Geometry: final body of the model. Coordinates: model frame, mm. Face numbers are marked on the shaded views. A direction names the side the tool comes from. Give positions to 0.01 mm unless a question says otherwise; leave off trailing zeros. Loops run counter-clockwise (first coordinate to the right, second up) from the corner with the lowest first, then second, coordinate; pieces in that order, holes last.
1. Section A-A, the plane y = 46. Output: boundary loops of the cut face in (x, z).
2. Section C-C, the plane x = -32. Output: boundary loops of the cut face in (y, z).
3. Section D-D, the plane y = 107.5. Output: boundary loops of the cut face in (x, z).
4. Material intervals for line 1 along Z through (x, y) = (-13, 172.5); line 2 along X through (y, z) = (112.5, -81.5); line 3 along Z through (x, y) = (-80, 21), sorted ascending.
5. Section B-B, the plane z = 82.5. Output: boundary loops of the cut face in (x, y).
6. First-contact query: P1, Ø0.9, axis at x = -177, y = 159, coming from the -Z side; P2, Ø6, axis at x = -83.5, y = 184.5, coming from the +Z side; P3, Ø19.5, axis at y = 148, z = -138, coming from the +X side; P4, Ø10, axis at x = -91.5, z = 80.5, coming from the -Y side. Flat tips, straight axial feed; report the tip coordinate or a pass-through.
7. Access query for the marked faces 1, 2, 3 and 4. Directions: +Z, -Z, +X, -X, +Y, -Y. A direction counts if a zero-diameter tool reaches every point of the face in a straight line with its end or side. Return the directions, or none.
Autodesk Inventor part; units mm, degrees
ref_plane "YZ Plane" through (0, 0, 0) normal (1, 0, 0) x (0, 1, 0)
ref_plane "XZ Plane" through (0, 0, 0) normal (0, 1, 0) x (-1, 0, 0)
ref_plane "XY Plane" through (0, 0, 0) normal (0, 0, 1) x (1, 0, 0)
sketch "Sketch1" plane through (0, 0, 0) normal (0, 1, 0) x (-1, 0, 0)
  line L0 (0, 213.3361) -> (190.5, 213.3361)
  line L1 (190.5, 213.3361) -> (190.5, -167.6639)
  line L2 (190.5, -167.6639) -> (0, -167.6639)
  line L3 (0, -167.6639) -> (0, 213.3361)
  point P0 (0, 0)
  dimension "d0" = 190.5
  dimension "d1" = 381
extrude "Extrusion1" add sketch "Sketch1" along normal blind 12.7
sketch "Sketch2" plane through (0, 12.7, 0) normal (0, 1, 0) x (1, 0, 0)
  line L0 (0, -213.3361) -> (-190.5, -213.3361)
  line L1 (-190.5, -213.3361) -> (-190.5, 167.6639)
  line L2 (-190.5, 167.6639) -> (0, 167.6639)
  line L3 (0, 167.6639) -> (0, -213.3361)
  line L4 (-177.8, 154.9639) -> (-177.8, -200.6361)
  line L5 (-177.8, -200.6361) -> (-12.7, -200.6361)
  line L6 (-12.7, -200.6361) -> (-12.7, 154.9639)
  line L7 (-12.7, 154.9639) -> (-177.8, 154.9639)
  line L8 (-177.0062, -199.8424) -> (-177.0062, 154.1701)
  line L9 (-177.0062, 154.1701) -> (-13.4938, 154.1701)
  line L10 (-13.4938, 154.1701) -> (-13.4938, -199.8424)
  line L11 (-13.4938, -199.8424) -> (-177.0062, -199.8424)
  point P0 (0, 0)
  dimension "d4" = 12.7
  dimension "d5" = 0.7937
extrude "Extrusion2" add sketch "Sketch2" along normal blind 203.2 contours L7 L6 L5 L4
sketch "Sketch3" plane through (-12.7, 12.7, 200.6361) normal (1, 0, 0) x (0, 0, -1)
  line L0 (354.8062, 203.2) -> (265.9062, 203.2)
  line L1 (265.9062, 203.2) -> (265.9062, 0)
  line L2 (265.9062, 0) -> (354.8062, 0)
  line L3 (354.8062, 0) -> (354.8062, 203.2)
  line L4 (354.8062, 0) -> (0.7938, 0)
  line L5 (0.7938, 203.2) -> (89.6938, 203.2)
  line L6 (89.6938, 203.2) -> (89.6938, 0)
  line L7 (89.6938, 0) -> (0.7938, 0)
  line L8 (0.7938, 0) -> (0.7938, 203.2)
  line L9 (89.6938, 203.2) -> (265.9062, 203.2)
  line L10 (265.9062, 203.2) -> (265.9062, 0)
  line L11 (265.9062, 0) -> (89.6938, 0)
  line L12 (89.6938, 0) -> (89.6938, 203.2)
  point P0 (200.6361, -12.7)
  point P1 (0, 203.2)
  dimension "d9" = 88.9
  dimension "d10" = 88.9
extrude "Extrusion3" cut sketch "Sketch3" against normal blind 50.8 contours L1 L4 L6 L9
sketch "Sketch4" plane through (-177.0062, 12.7, 199.8424) normal (1, 0, 0) x (0, 0, -1)
  line L0 (265.1125, 0) -> (265.1125, 203.2)
  line L1 (88.9, 0) -> (265.1125, 0)
  line L2 (265.1125, 0) -> (265.1125, 50.8)
  line L3 (265.1125, 50.8) -> (88.9, 50.8)
  line L4 (88.9, 50.8) -> (88.9, 0)
  line L5 (88.9, 203.2) -> (265.1125, 203.2)
  line L6 (265.1125, 203.2) -> (265.1125, 114.3)
  line L7 (265.1125, 114.3) -> (88.9, 114.3)
  line L8 (88.9, 114.3) -> (88.9, 203.2)
  point P0 (199.8424, -12.7)
  dimension "d13" = 50.8
  dimension "d14" = 88.9
extrude "Extrusion4" cut sketch "Sketch4" against normal blind 50.8
sketch "Sketch5" plane through (-177.8, 12.7, 200.6361) normal (-1, 0, 0) x (0, 0, 1)
  line L0 (-265.9062, 114.3) -> (-265.9062, 203.2)
  line L1 (-355.6, 0) -> (-355.6, 203.2)
  line L2 (-368.3, 0) -> (12.7, 0)
  line L3 (-355.6, 203.2) -> (-330.2, 203.2)
  line L4 (-330.2, 203.2) -> (-330.2, 0)
  line L5 (-330.2, 0) -> (-355.6, 0)
  line L6 (-355.6, 0) -> (-355.6, 203.2)
  line L7 (-265.9062, 203.2) -> (-291.3062, 203.2)
  line L8 (-291.3062, 203.2) -> (-291.3062, 0)
  line L9 (-291.3062, 0) -> (-265.9062, 0)
  line L10 (-265.9062, 0) -> (-265.9062, 203.2)
  line L11 (-330.2, 203.2) -> (-291.3062, 203.2)
  line L12 (-291.3062, 203.2) -> (-291.3062, 0)
  line L13 (-291.3062, 0) -> (-330.2, 0)
  line L14 (-330.2, 0) -> (-330.2, 203.2)
  point P0 (-200.6361, -12.7)
  dimension "d17" = 89.6937
  dimension "d18" = 25.4
  dimension "d19" = 25.4
extrude "Extrusion5" cut sketch "Sketch5" against normal blind 25.4 contours L8 L2 L4 L11
sketch "Sketch6" plane through (-177.8, 12.7, 200.6361) normal (-1, 0, 0) x (0, 0, 1)
  line L0 (-89.6938, 114.3) -> (-265.9062, 114.3)
  line L1 (0, 0) -> (-89.6938, 0)
  line L2 (0, 203.2) -> (-25.4, 203.2)
  line L3 (-25.4, 203.2) -> (-25.4, 0)
  line L4 (-25.4, 0) -> (0, 0)
  line L5 (0, 0) -> (0, 203.2)
  line L6 (-89.6938, 203.2) -> (0, 203.2)
  line L7 (-89.6938, 0) -> (-64.2938, 0)
  line L8 (-64.2938, 0) -> (-64.2938, 203.2)
  line L9 (-64.2938, 203.2) -> (-89.6938, 203.2)
  line L10 (-89.6938, 203.2) -> (-89.6938, 0)
  line L11 (-64.2938, 203.2) -> (-25.4, 203.2)
  line L12 (-25.4, 203.2) -> (-25.4, 0)
  line L13 (-25.4, 0) -> (-64.2938, 0)
  line L14 (-64.2938, 0) -> (-64.2938, 203.2)
  line L15 (-64.2938, 203.2) -> (-25.4, 203.2)
  line L16 (-25.4, 203.2) -> (-25.4, 0)
  line L17 (-25.4, 0) -> (-64.2938, 0)
  line L18 (-64.2938, 0) -> (-64.2938, 203.2)
  point P0 (-200.6361, -12.7)
  dimension "d22" = 25.4
  dimension "d23" = 25.4
extrude "Extrusion6" cut sketch "Sketch6" against normal blind 25.4 contours L1 L8 L6 L3
properties part number "soccer_goal.ipj"
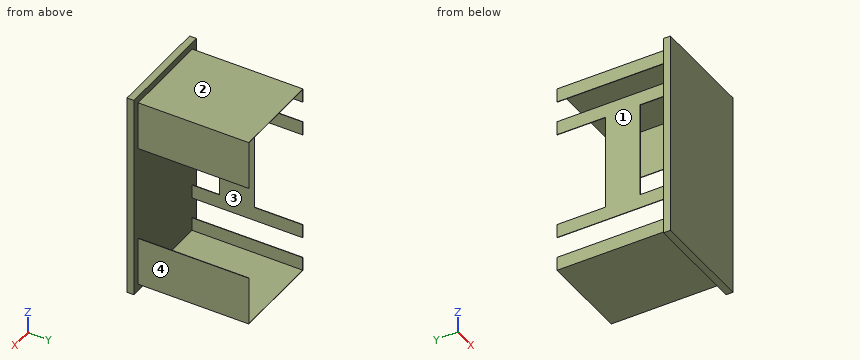
Answers below:
1. outline: (-177.8, -154.96) - (-12.7, -154.96) - (-12.7, -65.27) - (-13.49, -65.27) - (-13.49, -154.17) - (-177.01, -154.17) - (-177.01, -129.56) - (-177.8, -129.56) - close; (-177.8, -90.67) - (-177.01, -90.67) - (-177.01, -65.27) - (-177.8, -65.27) - close; (-177.8, 110.94) - (-177.01, 110.94) - (-177.01, 136.34) - (-177.8, 136.34) - close; (-177.8, 175.24) - (-177.01, 175.24) - (-177.01, 199.84) - (-13.49, 199.84) - (-13.49, 110.94) - (-12.7, 110.94) - (-12.7, 200.64) - (-177.8, 200.64) - close
2. outline: (0, -167.66) - (12.7, -167.66) - (12.7, -154.96) - (215.9, -154.96) - (215.9, -154.17) - (12.7, -154.17) - (12.7, 199.84) - (215.9, 199.84) - (215.9, 200.64) - (12.7, 200.64) - (12.7, 213.34) - (0, 213.34) - close
3. outline: (-177.8, -154.96) - (-12.7, -154.96) - (-12.7, -65.27) - (-13.49, -65.27) - (-13.49, -154.17) - (-177.01, -154.17) - (-177.01, -129.56) - (-177.8, -129.56) - close; (-177.8, -90.67) - (-177.01, -90.67) - (-177.01, 136.34) - (-177.8, 136.34) - close; (-177.8, 175.24) - (-177.01, 175.24) - (-177.01, 199.84) - (-13.49, 199.84) - (-13.49, 110.94) - (-12.7, 110.94) - (-12.7, 200.64) - (-177.8, 200.64) - close
4. line 1: z = -154.96 to -65.27, 110.94 to 200.64
4. line 2: x = -177.8 to -177.01, -13.49 to -12.7
4. line 3: z = -154.96 to -154.17, 199.84 to 200.64
5. outline: (-190.5, 0) - (0, 0) - (0, 12.7) - (-190.5, 12.7) - close; (-177.8, 63.5) - (-177.01, 63.5) - (-177.01, 127) - (-177.8, 127) - close
6. P1: stops at z = -154.96
6. P2: stops at z = 200.64
6. P3: stops at x = -12.7
6. P4: stops at y = 0
7. face 1: +Z, -Z, -X, +Y
7. face 2: +Z, +X, -X, +Y
7. face 3: +Y
7. face 4: +Z, -Z, +X, +Y
